```python
from build123d import *

# Parameters (mm, degrees)
SKETCH027_W     = 98
SKETCH027_H     = 59
PAD014_DEPTH    = 25
SKETCH028_W     = 95
SKETCH028_H     = 56
POCKET008_DEPTH = 22
SKETCH029_W     = 56
SKETCH029_H     = 2
PAD015_DEPTH    = 1
SKETCH030_W     = 56.025157
SKETCH030_H     = 2
PAD016_DEPTH    = 1
SKETCH031_R     = 1.75
PAD017_DEPTH    = 2
SKETCH032_R     = 0.95
POCKET009_DEPTH = 3
FILLET003_R     = 1.9
POCKET010_DEPTH = 3
FILLET004_R     = 1


with BuildPart() as part:
    # Sketch027 → Pad014 (new body)
    with BuildSketch(Plane.XY):
        Rectangle(SKETCH027_W, SKETCH027_H)
    extrude(amount=PAD014_DEPTH)

    # Sketch028 (on Face6 of Pad014) → Pocket008 (cut)
    with BuildSketch(Plane.XY.offset(25)):
        Rectangle(SKETCH028_W, SKETCH028_H)
    extrude(amount=-POCKET008_DEPTH, mode=Mode.SUBTRACT)

    # Sketch029 (on Face9 of Pocket008) → Pad015 (join)
    with BuildSketch(Plane.YZ.offset(-47.5)):
        with Locations((0, 14.5)):
            Rectangle(SKETCH029_W, SKETCH029_H)
    extrude(amount=PAD015_DEPTH)

    # Sketch030 (on Face7 of Pad015) → Pad016 (join)
    with BuildSketch(Plane(origin=(47.5, 0, 0), x_dir=(0, -1, 0), z_dir=(-1, 0, 0))):
        with Locations((0.0125785, 14.5)):
            Rectangle(SKETCH030_W, SKETCH030_H)
    extrude(amount=PAD016_DEPTH)

    # Sketch031 (on Face16 of Pad016) → Pad017 (join)
    with BuildSketch(Plane.XY.offset(3)):
        with Locations((-2, -10.78)):
            Circle(SKETCH031_R)
        with Locations((45, -10.78)):
            Circle(SKETCH031_R)
        with Locations((45, -22.21)):
            Circle(SKETCH031_R)
        with Locations((-2, -22.21)):
            Circle(SKETCH031_R)
    extrude(amount=PAD017_DEPTH)

    # Sketch032 (on Face26 of Pad017) → Pocket009 (cut)
    with BuildSketch(Plane.XY.offset(5)):
        with Locations((-2.01, -10.76)):
            Circle(SKETCH032_R)
        with Locations((-2.01, -22.21)):
            Circle(SKETCH032_R)
        with Locations((44.95, -22.21)):
            Circle(SKETCH032_R)
        with Locations((44.95, -10.76)):
            Circle(SKETCH032_R)
    extrude(amount=-POCKET009_DEPTH, mode=Mode.SUBTRACT)

    # Fillet003
    fillet003_edges = [part.edges().sort_by_distance(p)[0] for p in [
        (-3.75, -10.78, 3),
        (-3.75, -22.21, 3),
        (43.25, -10.78, 3),
        (43.25, -22.21, 3),
    ]]
    fillet(fillet003_edges, radius=FILLET003_R)

    # Sketch033 (on Face2 of Fillet003) → Pocket010 (cut)
    with BuildSketch(Plane(origin=(47.5, 0, 0), x_dir=(0, -1, 0), z_dir=(-1, 0, 0))):
        with BuildLine():
            Line((8.293246951, 7.809269951), (8.293246951, 7.783904049))
            ThreePointArc((8.293246951, 7.783904049), (9.1682118571, 5.6715519061), (11.280564, 4.796587))
            Line((11.280564, 4.796587), (21.280564, 4.796587))
            ThreePointArc((21.280564, 4.796587), (23.3929161429, 5.6715519061), (24.267881049, 7.783904049))
            Line((24.267881049, 7.783904049), (24.267881049, 7.809269951))
            ThreePointArc((24.267881049, 7.809269951), (23.3929161429, 9.9216220939), (21.280564, 10.796587))
            Line((21.280564, 10.796587), (11.280564, 10.796587))
            ThreePointArc((11.280564, 10.796587), (9.1682118571, 9.9216220939), (8.293246951, 7.809269951))
        make_face()
    extrude(amount=-POCKET010_DEPTH, mode=Mode.SUBTRACT)

    # Fillet004
    fillet004_edges = [part.edges().sort_by_distance(p)[0] for p in [
        (49, -9.168212, 9.921622),
        (49, -9.168212, 5.671552),
        (49, -16.280564, 4.796587),
        (49, -16.280564, 10.796587),
        (49, -23.392916, 9.921622),
        (49, -23.392916, 5.671552),
    ]]
    fillet(fillet004_edges, radius=FILLET004_R)


solid = part.part
```
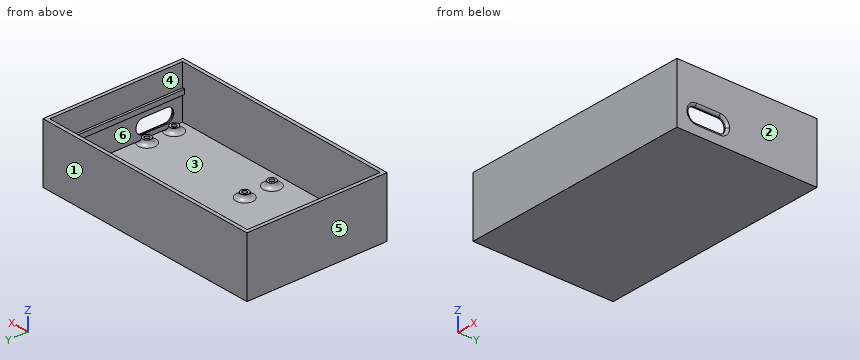
Part model, mm, in its own coordinate system. Face numbers are marked on the shaded views. A direction names the side the tool comes from. Give positions to 0.01 mm unless a question says otherwise; leave off trailing zeros. Write each loop counter-clockwise with the first axis right and the second up, starting at its lowest first coordinate (ties: lowest second). Pieces come first, ordered by that corner, then holes. Notation, with made-up numbers: M 74,19.5 L 112,19.5 A32 cw 112,52.5 Z; hole C 10.5,65.25 d6. An arc over 180 degrees is marked long. Use CSV: the item, a comma, the result in double quotes.
Item 1: Which spindle directions (+Z, -Z, +X, -X, +Y, -Y) get a long thin tool onto all of the face, cutting with end or side? Do the marked faces 4, 5 and 6. Say none if no direction does.
Taken from the geometry:
face 4,"+Z"
face 5,"+Z, -Z, -X, +Y, -Y"
face 6,"none"
Item 2: Pin check, flat tips, straight feed: P1, Ø8, axis at y = -22, z = 6.5, coming from the +X side; P2, Ø1.8, axis at x = 45.5, y = -11, coming from the +Z side. Stop position of each tip, or through.
Taken from the geometry:
P1,"stops at x = 49"
P2,"stops at z = 5"
Item 3: Slice it at C-C on x = -2. Write the cut outline in (y, z), plus the area to 3 significant figures.
Taken from the geometry:
outline,"M -29.5,0 L 29.5,0 L 29.5,25 L 28,25 L 28,3 L -7.13,3 A1.9 cw -9.03,4.9 L -9.03,5 L -9.81,5 L -9.81,2 L -11.71,2 L -11.71,5 L -12.53,5 L -12.53,4.9 A1.9 cw -14.43,3 L -18.56,3 A1.9 cw -20.46,4.9 L -20.46,5 L -21.26,5 L -21.26,2 L -23.16,2 L -23.16,5 L -23.96,5 L -23.96,4.9 A1.9 cw -25.86,3 L -28,3 L -28,25 L -29.5,25 Z"
area,"249 mm²"
Item 4: Slice it at B-B on x = 13. Write the cut outline in (y, z).
Taken from the geometry:
outline,"M -29.5,0 L 29.5,0 L 29.5,25 L 28,25 L 28,3 L -28,3 L -28,25 L -29.5,25 Z"
Item 5: Drill centre lines: probe 1 along Y at (x, z) = (44.95, 2.85); probe 2 along X at (y, z) = (15, 22.25); probe 3 along Y at (x, z) = (-9, 23.25). Where is each one in solid material? Low to high.
Taken from the geometry:
probe 1,"y = -29.5 to -23.16, -21.26 to -11.71, -9.81 to 29.5"
probe 2,"x = -49 to -47.5, 47.5 to 49"
probe 3,"y = -29.5 to -28, 28 to 29.5"
Item 6: Pull direction Y, two halves, no side cores. Call the marked faces 1, 2 and 3: +Y half, -Y half, draft (parallel to the pull), parting line (faces both ways), or undercut.
Taken from the geometry:
face 1,"+Y half"
face 2,"draft"
face 3,"undercut"
Item 7: Slice it at A-A on y = 15.5. Write the cut outline in (x, z).
Taken from the geometry:
outline,"M -49,0 L 49,0 L 49,25 L 47.5,25 L 47.5,15.5 L 46.5,15.5 L 46.5,13.5 L 47.5,13.5 L 47.5,3 L -47.5,3 L -47.5,13.5 L -46.5,13.5 L -46.5,15.5 L -47.5,15.5 L -47.5,25 L -49,25 Z"
